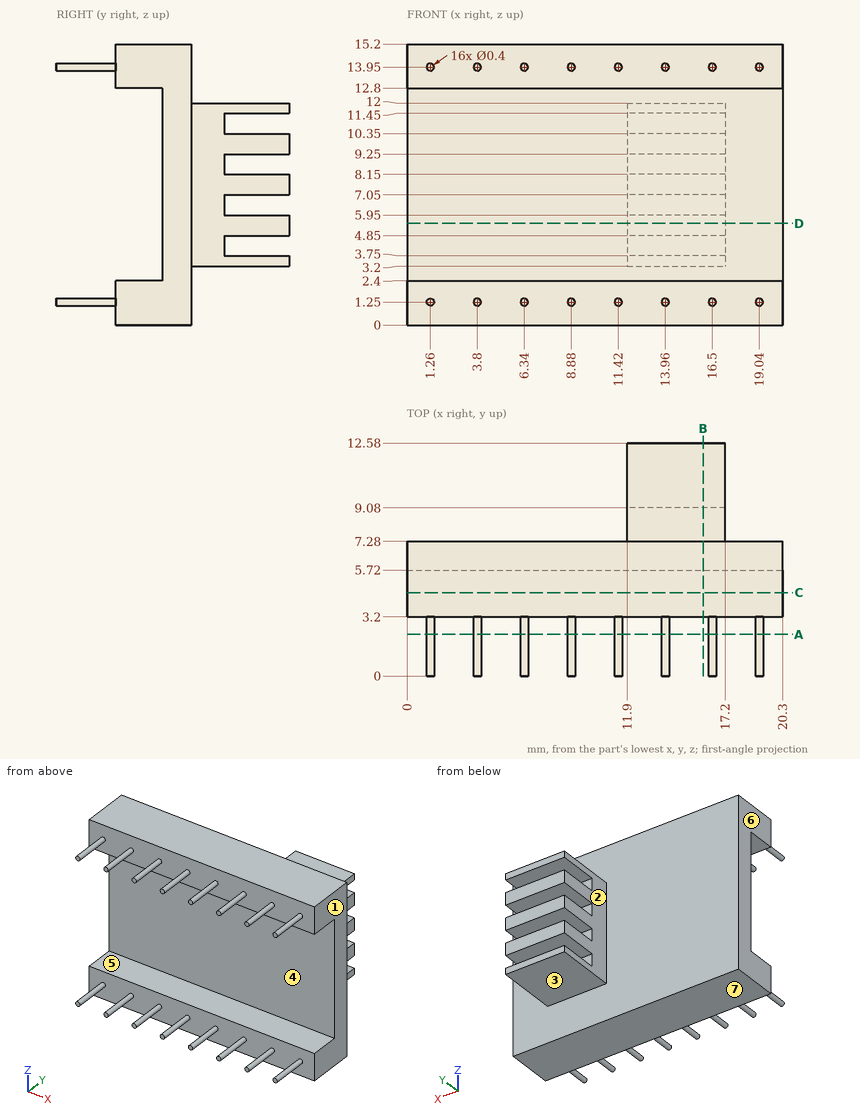
Design review of the part shown in the three views and the two pictorial views. Dimensions are in mm from the part's minimum x, y and z. A direction names the side the tool comes from. Give positions to 0.01 mm unless a question says otherwise; leave off trailing zeros. Write each loop counter-clockwise with the first axis right and the second up, starting at its lowest first coordinate (ties: lowest second). Pieces come first, ordered by that corner, then holes.
Item 1: Take a section at B-B (x = 16). Give the boundary of the cut face in (y, z), and give its area (3 significant figures).
Item 2: The part is to be moulded in two halves that separate along Z. For the marked faces 5, 6 and 7, say which applies: +Z half, -Z half, draft (parallel to the pull), parting line (faces both ways), or undercut.
Item 3: Insertion check: P1, Ø4, axis at x = 13.5, y = 11, coming from the +Z side; P2, Ø3, axis at x = 12, z = 8.5, coming from the -Y side; P3, Ø1.6, axis at x = 15, y = 9, coming from the -Z side. Each pin has a flat end and moves straight along its axis. Give the tip position at first contact, or say it passes through.
Item 4: Wall thickness on probe 1 along Z at (x, y) = (15.5, 10.25); probe 2 along Z at (x, y) = (7.5, 4.25); probe 3 along Z at (x, y) = (3.75, 2): over which ranges is each line inside the solid? List them lowest first.
Item 5: Machinability: for the marked faces 1, 2, 3 and 4, which of the approach directions +Z, -Z, +X, -X, +Y, -Y give a long, thin tool a straight path to every point of the face, cutting with its end or side? Answer none if there is none.
Item 6: Take a section at C-C (y = 4.5). Give the boundary of the cut face in (x, z), and give its area (3 significant figures).
Item 7: Take a section at D-D (z = 5.5). Give the boundary of the cut face in (x, y), and give its area (3 significant figures).
Item 8: Take a section at A-A (y = 2.25). Give the number of separate pieces and of enclosed holes in the cut face, and give its area (3 significant figures).
Established:
1. outline: (3.2, 0) - (7.28, 0) - (7.28, 3.2) - (12.58, 3.2) - (12.58, 3.75) - (9.08, 3.75) - (9.08, 4.85) - (12.58, 4.85) - (12.58, 5.95) - (9.08, 5.95) - (9.08, 7.05) - (12.58, 7.05) - (12.58, 8.15) - (9.08, 8.15) - (9.08, 9.25) - (12.58, 9.25) - (12.58, 10.35) - (9.08, 10.35) - (9.08, 11.45) - (12.58, 11.45) - (12.58, 12) - (7.28, 12) - (7.28, 15.2) - (3.2, 15.2) - (3.2, 12.8) - (5.72, 12.8) - (5.72, 2.4) - (3.2, 2.4) - close
1. area: 67.0 mm2
2. face 5: undercut
2. face 6: draft
2. face 7: -Z half
3. P1: stops at z = 12
3. P2: stops at y = 5.72
3. P3: stops at z = 3.2
4. probe 1: z = 3.2 to 3.75, 4.85 to 5.95, 7.05 to 8.15, 9.25 to 10.35, 11.45 to 12
4. probe 2: z = 0 to 2.4, 12.8 to 15.2
4. probe 3: z = 1.06 to 1.44, 13.76 to 14.14
5. face 1: +Z, -Z, +X, +Y, -Y
5. face 2: +Z, -Z, -X, +Y
5. face 3: -Z, +X, -X, +Y
5. face 4: +X, -X, -Y
6. outline: (0, 0) - (20.3, 0) - (20.3, 2.4) - (0, 2.4) - close; (0, 12.8) - (20.3, 12.8) - (20.3, 15.2) - (0, 15.2) - close
6. area: 97.4 mm2
7. outline: (0, 5.72) - (20.3, 5.72) - (20.3, 7.28) - (17.2, 7.28) - (17.2, 12.58) - (11.9, 12.58) - (11.9, 7.28) - (0, 7.28) - close
7. area: 59.8 mm2
8. separate pieces: 16
8. enclosed holes: 0
8. area: 2.01 mm2
